Autodesk Inventor part; units mm, degrees
ref_plane "YZ Plane" through (0, 0, 0) normal (1, 0, 0) x (0, 1, 0)
ref_plane "XZ Plane" through (0, 0, 0) normal (0, 1, 0) x (-1, 0, 0)
ref_plane "XY Plane" through (0, 0, 0) normal (0, 0, 1) x (1, 0, 0)
sketch "Sketch1" plane through (0, 0, 0) normal (0, 0, 1) x (1, 0, 0)
  line L0 (0, 0) -> (25.4, 0)
  line L1 (25.4, 0) -> (25.4, -50.8)
  line L2 (25.4, -50.8) -> (0, -50.8)
  line L3 (0, -50.8) -> (0, 0)
  line L4 (22.225, -3.175) -> (3.175, -3.175)
  line L5 (3.175, -3.175) -> (3.175, -47.625)
  line L6 (3.175, -47.625) -> (22.225, -47.625)
  line L7 (22.225, -47.625) -> (22.225, -3.175)
  dimension "d0" = 25.4
  dimension "d1" = 50.8
  dimension "d2" = 3.175
extrude "Extrusion1" add sketch "Sketch1" along normal blind 762
sketch "Sketch3" plane through (25.4, -50.8, 0) normal (1, 0, 0) x (0, 0, -1)
  circle A0 centre (-38.1, 25.4) radius 14.2875
  line L0 (0, 50.8) -> (0, 0)
  line L1 (0, 50.8) -> (-762, 50.8)
  dimension "d13" = 38.1
  dimension "d14" = 25.4
  dimension "d15" = 28.575
extrude "Extrusion3" cut sketch "Sketch3" against normal blind 25.4
sketch "Sketch4" plane through (25.4, -50.8, 0) normal (1, 0, 0) x (0, 0, -1)
  circle A0 centre (-723.9, 25.4) radius 14.2875
  circle A1 centre (-381, 25.4) radius 14.2875
  line L0 (-762, 0) -> (-762, 50.8)
  line L1 (0, 50.8) -> (-762, 50.8)
  circle A2 centre (-38.1, 25.4) radius 14.2875
  dimension "d19" = 38.1
  dimension "d20" = 25.4
  dimension "d21" = 28.575
  dimension "d22" = 25.4
  dimension "d23" = 28.575
  dimension "d26" = 342.9
  dimension "d27" = 342.9
extrude "Extrusion4" cut sketch "Sketch4" against normal blind 25.4 contours A0 | A1
properties part number "DRL short Angle"
For this review, take the finished solid that the model builds, in its own axes (mm). A direction names the side the tool comes from. Coordinates: 2 decimals unless noted, no trailing zeros. Loops run counter-clockwise (first coordinate to the right, second up) from the corner with the lowest first, then second, coordinate; pieces in that order, holes last.
1. Mouldability with a two-part tool opening along X and no side actions: class faces 3 (the flat face through (2, -27, 762)), 4 (the flat face through (25.4, -42, 376)), 5 (the flat face through (22.225, -41, 376)) as +X half, -X half, draft (parallel to the pull), parting line (faces both ways), or undercut.
2. Add section C-C, the plane z = 143. Give the boundary of the cut face in (x, y) (3 decimals), then the cut area to 3 significant figures.
3. For faces 1 (the flat face through (13, -3.175, 376)), 2 (the flat face through (0, -9, 376)), list the 3-axis set-ups (+Z, -Z, +X, -X, +Y, -Y) from which the entire face can be reached by the end or side of a thin tool; tool diameter is ignored.
4. Add section B-B, the plane y = -25.4. Count the separate pieces of the cut face and the enclosed holes in it, then the cut area to 3 significant figures.
5. Insertion check: P1, Ø1, axis at x = 20.5, z = 607.5, coming from the +Y side. The pin has a flat end and moves straight along its axis. Give the tip position at first contact, or say it passes through.
6. Add section A-A, the plane z = 381. Give the boundary of the cut face in (x, y) (1 decimal), then the cut area to 3 significant figures.
7. For line 1 (X direction, y = -17.5, z = 126.5) (3 decimals); line 2 (Y direction, x = 6.5, z = 232) (3 decimals); line 3 (Y direction, x = 2.25, z = 381), list the stretches that pass through material, from the lowest coordinate up.
Result:
1. face 3: draft
1. face 4: +X half
1. face 5: undercut
2. outline: (0, -50.8) - (25.4, -50.8) - (25.4, 0) - (0, 0) - close; hole (3.175, -47.625) - (22.225, -47.625) - (22.225, -3.175) - (3.175, -3.175) - close
2. area: 444 mm2
3. face 1: +Z, -Z
3. face 2: +Z, -Z, -X, +Y, -Y
4. separate pieces: 8
4. enclosed holes: 0
4. area: 4,290 mm2
5. P1: stops at y = 0
6. outline: (0, -50.8) - (25.4, -50.8) - (25.4, -39.7) - (22.2, -39.7) - (22.2, -47.6) - (3.2, -47.6) - (3.2, -39.7) - (0, -39.7) - close; (0, -11.1) - (3.2, -11.1) - (3.2, -3.2) - (22.2, -3.2) - (22.2, -11.1) - (25.4, -11.1) - (25.4, 0) - (0, 0) - close
6. area: 262 mm2
7. line 1: x = 0 to 3.175, 22.225 to 25.4
7. line 2: y = -50.8 to -47.625, -3.175 to 0
7. line 3: y = -50.8 to -39.69, -11.11 to 0
